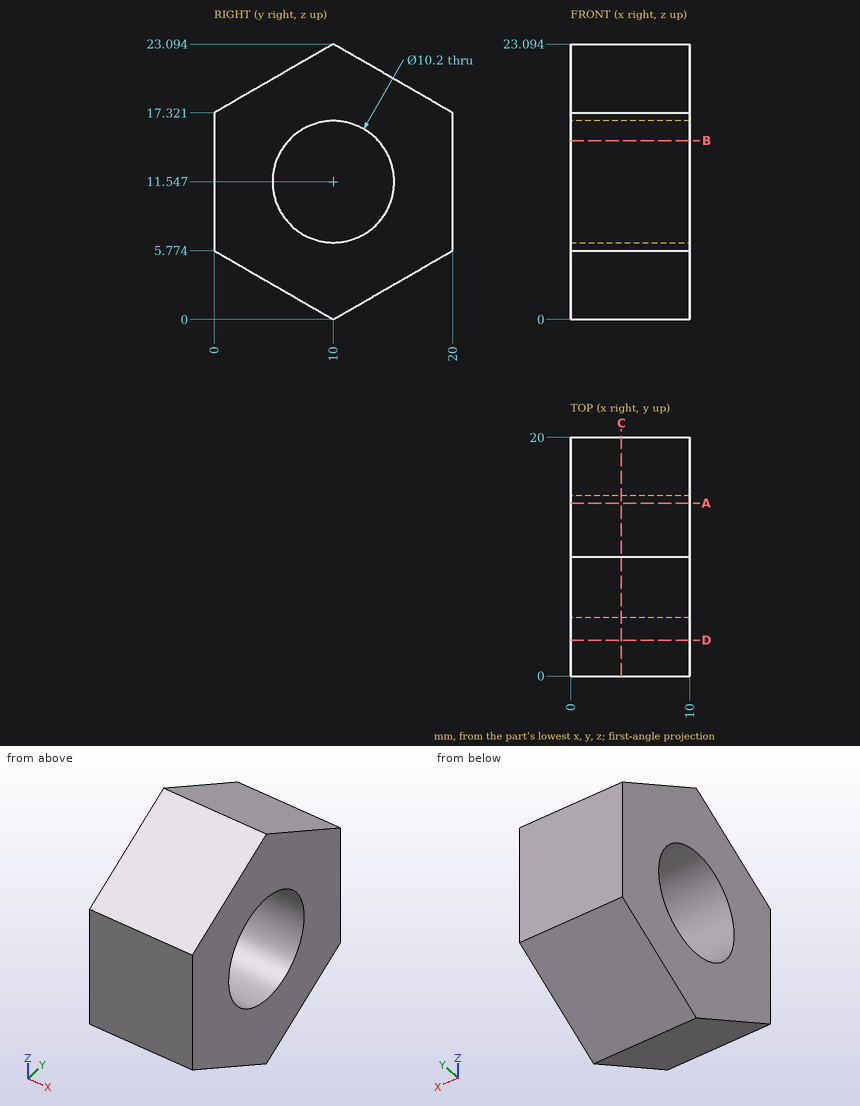
Here's the drawing with two shaded views (mm, measured from the low corner). I have some questions. Coordinates: 2 decimals unless noted, no trailing zeros. Order: outer loops, then holes, each group sorted by start corner. A loop starts at its lowest first (then second) coordinate and runs counter-clockwise, first axis right, second up.
Item 1: If we section it at B-B, the plane z = 15: List the corners of the cut face in (x, y) for me.
Response values:
outline: (0, 0) - (10, 0) - (10, 6.25) - (0, 6.25) - close; (0, 13.75) - (10, 13.75) - (10, 20) - (0, 20) - close
Item 2: If we section it at D-D, the plane y = 3: List the corners of the cut face in (x, z) for me.
Response values:
outline: (0, 4.04) - (10, 4.04) - (10, 19.05) - (0, 19.05) - close
Item 3: If we section it at A-A, the plane y = 14.5: List the corners of the cut face in (x, z) for me (1 decimal).
Response values:
outline: (0, 2.6) - (10, 2.6) - (10, 9.1) - (0, 9.1) - close; (0, 13.9) - (10, 13.9) - (10, 20.5) - (0, 20.5) - close
Item 4: I need wall thicknesses on probe 1 along Y at (x, z) = (4.5, 8.75) (1 decimal); probe 2 along Y at (x, z) = (3, 9.5); probe 3 along Z at (x, y) = (7.75, 13.5) (1 decimal). Which ranges of each line are inside material? Lowest first, please.
Response values:
probe 1: y = 0 to 5.7, 14.3 to 20
probe 2: y = 0 to 5.33, 14.67 to 20
probe 3: z = 2 to 7.8, 15.3 to 21.1
Item 5: I'm going to push flat-ended pins straight in: pin 1 Ø1.5 at (x, z) = (7.5, 18) entering from +Y; pin 2 Ø1.5 at (x, y) = (9, 8) entering from -Z; pin 3 Ø1.5 at (x, y) = (6.5, 8) entering from +Z; pin 4 Ø1.5 at (x, y) = (7, 11.5) entering from -Z. Where does each tip first touch, or does it pass through?
Response values:
pin 1: stops at y = 20
pin 2: stops at z = 0.72
pin 3: stops at z = 22.37
pin 4: stops at z = 0.43
Item 6: If we section it at C-C, the plane x = 4.25: List the corners of the cut face in (y, z) for me (1 decimal).
Response values:
outline: (0, 5.8) - (10, 0) - (20, 5.8) - (20, 17.3) - (10, 23.1) - (0, 17.3) - close; hole circle Ø10.2 at (10, 11.5)
